Can you work these out from the model? Positions are in its coordinate system, mm. A direction names the side the tool comes from. Give positions to 0.01 mm unless a question says otherwise; leave off trailing zeros. Loops run counter-clockwise (first coordinate to the right, second up) from the corner with the lowest first, then second, coordinate; pieces in that order, holes last. Notation, with made-up numbers: M 15.5,71 L 22.5,71 A14 ccw 22.5,82 Z; hole C -36.75,8 d7. An arc over 180 degrees is marked long. Use CSV: the item, a comma, the result in double quotes.
from build123d import *

# Parameters (mm, degrees)
F0_R     = 15
F2_DEPTH = 5
F1_R     = 1.1
F3_DEPTH = 5
F4_DEPTH = 5
F5_R     = 11.75
F6_DEPTH = 5
F7_R     = 11
F8_DEPTH = 10


with BuildPart() as f2:
    # F0 (on Front) → F2 (new body)
    with BuildSketch(Plane.XZ):
        Circle(F0_R)
    extrude(amount=-F2_DEPTH)

    # F1 (on Front) → F3 (cut)
    with BuildSketch(Plane.XZ):
        with Locations((-13.25, 0)):
            Circle(F1_R)
    extrude(amount=-F3_DEPTH, mode=Mode.SUBTRACT)

    # F1 (on Front) → F4 (cut)
    with BuildSketch(Plane.XZ):
        with Locations((-13.25, 0)):
            Circle(F1_R)
        with Locations((13.25, 0.028307)):
            Circle(F1_R)
    extrude(amount=-F4_DEPTH, mode=Mode.SUBTRACT)

    # F5 (on face) → F6 (join)
    with BuildSketch(Plane.XZ):
        Circle(F5_R)
    extrude(amount=F6_DEPTH)

    # F7 (on face) → F8 (cut)
    with BuildSketch(Plane.XZ.offset(5)):
        Circle(F7_R)
    extrude(amount=-F8_DEPTH, mode=Mode.SUBTRACT)


solid = f2.part
Q1. For faces 1 (the cylindrical face through (11.207, -2.465, 3.529)), 2 (the cylindrical face through (12.377, 2.465, -0.641)), which set-ups out of +Z, -Z, +X, -X, +Y, -Y let a thin tool reach every point of the face, with its end or its side?
Model answer:
face 1,"-Y"
face 2,"+Y, -Y"
Q2. I want a section at D-D, the plane x = 13.25. Please give me the cut outline in (y, z), then the cut area to 3 significant figures.
Model answer:
outline,"M 0,-7.03 L 5,-7.03 L 5,-1.07 L 0,-1.07 Z; M 0,1.13 L 5,1.13 L 5,7.03 L 0,7.03 Z"
area,"59.3 mm2"
Q3. I'm going to push flat-ended pins straight in: P1, Ø1, axis at x = 11, y = 0.5, coming from the -Z side; P2, Ø3, axis at x = -3.5, y = 2.5, coming from the -Z side; P3, Ø3, axis at x = 13.25, z = 0.03, coming from the +Y side; P4, Ø3, axis at y = 1.5, z = 4.5, coming from the +X side. Where does each tip first touch, or does it pass through?
Model answer:
P1,"z = -10.71"
P2,"z = -14.87"
P3,"y = 5"
P4,"x = 14.7"
Q4. If we mould it in two halves opening along X, with no side actions, what happens to faces 3 (the cylindrical face through (-14.985, 2.465, 0.66)), 4 (the cylindrical face through (-14.35, 2.46, 0.05)), 5 (the flat face through (-9, 0, 8))? For each: released by +X, released by -X, zero draft, split by the parting line, or undercut.
Model answer:
face 3,"split by the parting line"
face 4,"undercut"
face 5,"zero draft"
Q5. I want a section at C-C, the plane y = -4.5. Please give me the cut outline in (x, z).
Model answer:
outline,"C 0,0 d23.5; hole C 0,0 d22"
Q6. Please list where these lines run through material, in increasing order: L1, parallel to Z at x = -4, y = 2.5; L2, parallel to X at y = -3, z = -3.25; L3, parallel to Z at x = -7, y = -1.5. Write a range as from..to.
Model answer:
L1,"-14.46..-10.25, 10.25..14.46"
L2,"-11.29..-10.51, 10.51..11.29"
L3,"-9.44..-8.49, 8.49..9.44"
Q7. I want a section at A-A, the plane x = 0. Please give me the cut outline in (y, z), then the cut area to 3 significant figures.
Model answer:
outline,"M -5,-11.75 L 0,-11.75 L 0,-15 L 5,-15 L 5,-11 L -5,-11 Z; M -5,11 L 5,11 L 5,15 L 0,15 L 0,11.75 L -5,11.75 Z"
area,"47.5 mm2"
Q8. I want a section at B-B, the plane z = -7.5. Please give me the cut outline in (x, y).
Model answer:
outline,"M -12.99,0 L -9.05,0 L -9.05,-5 L -8.05,-5 L -8.05,5 L -12.99,5 Z; M 8.05,-5 L 9.05,-5 L 9.05,0 L 12.99,0 L 12.99,5 L 8.05,5 Z"
